Check sheet for the modelled part. Datum: model origin and axes. Units: mm. A direction names the side the tool comes from. Round coordinates to 2 decimals unless told otherwise and drop trailing zeros. Write each loop counter-clockwise with the first axis right and the second up, starting at its lowest first coordinate (ties: lowest second). Pieces come first, ordered by that corner, then holes.
Item 1: Depth check by flat-ended pin: pin 1 (12 mm diameter, centred on y = 15.5, z = 22.5, fed in from -X); pin 2 (8 mm diameter, centred on y = -33.5, z = 21, fed in from +X); pin 3 (3 mm diameter, centred on x = 19, y = 0.5, fed in from -Z). Enter the tip coordinate at first touch or a pass-through.
Item 2: Set-up check for faces 1 (the flat face through (-50, 35, 30)), 2 (the cylindrical face through (-27.5, 0.1, 4.9)), 3 (the cylindrical face through (-57.15, 36.99, 25.35)), 4 (the flat face through (-60, 0, 5)), 5 (the flat face through (-24, -1, 10)): record each of +Z, -Z, +X, -X, +Y, -Y from which the full face is reachable in a straight line by a thin tool's end or side.
Item 3: Section check A-A, the plane z = 35. State how many separate pieces and enclosed holes the cut face has, plus the area to 3 significant figures.
Item 4: Section check B-B, the plane x = -21.5. Record the cut outline in (y, z), plus the area to 3 significant figures.
Item 5: Section check C-C, the plane y = 0. Record the cut outline in (x, z).
Item 6: Release check for a two-part mould opening along Y. For faces 6 (the cylindrical face through (-57.15, -36.99, 25.35)), 7 (the flat face through (70, -1, 52)), 8 (the flat face through (-55, 30, 30)) record: pulls with the +Y half, pulls with the -Y half, needs draft (parallel to the pull), parting line crosses it, or undercut.
Item 7: Material ranges on line 1 along Z through (x, y) = (-19, -14); line 2 along Y through (x, z) = (-30, 8); line 3 along Z through (x, y) = (60.5, 37.5), recorded low to high.
Item 8: Section check D-D, the plane y = -36.5. Record the cut outline in (x, z).
from build123d import *

# Parameters (mm, degrees)
SALIENTE_EXTRUIR2_DEPTH = 50
CROQUIS4_W              = 140
CROQUIS4_H              = 100
SALIENTE_EXTRUIR3_DEPTH = 5
CROQUIS5_R              = 5
CORTAR_EXTRUIR1_DEPTH   = 5
CROQUIS6_W              = 50
CROQUIS6_H              = 40
CORTAR_EXTRUIR2_DEPTH   = 80
CROQUIS7_W              = 40
CROQUIS7_H              = 60
CORTAR_EXTRUIR3_DEPTH   = 50
CROQUIS8_R              = 2.5
CORTAR_EXTRUIR5_DEPTH   = 20
REDONDEO1_R             = 10
REDONDEO2_R             = 10
REDONDEO3_R             = 10
REDONDEO4_R             = 10


with BuildPart() as part:
    # Croquis1 → Saliente-Extruir2 (new body)
    with BuildSketch(Plane.XY):
        with BuildLine():
            Line((-60, 40), (-60, -40))
            Line((-60, -40), (20.000000086, -40))
            ThreePointArc((20.000000086, -40), (60, 8.6e-08), (19.999999914, 40))
            Line((19.999999914, 40), (-60, 40))
        make_face()
    extrude(amount=SALIENTE_EXTRUIR2_DEPTH)

    # Croquis4 → Saliente-Extruir3 (add)
    with BuildSketch(Plane.XY.offset(50)):
        Rectangle(CROQUIS4_W, CROQUIS4_H)
    extrude(amount=SALIENTE_EXTRUIR3_DEPTH)

    # Croquis5 → Cortar-Extruir1 (cut)
    with BuildSketch(Plane(origin=(0, 0, 0), x_dir=(-1, 0, 0), z_dir=(0, 0, -1))):
        with Locations((-20, 0)):
            Circle(CROQUIS5_R)
    extrude(amount=-CORTAR_EXTRUIR1_DEPTH, mode=Mode.SUBTRACT)

    # Croquis6 → Cortar-Extruir2 (cut)
    with BuildSketch(Plane(origin=(0, 40, 0), x_dir=(1, 0, 0), z_dir=(0, 1, 0))):
        with Locations((-25, -30)):
            Rectangle(CROQUIS6_W, CROQUIS6_H)
    extrude(amount=-CORTAR_EXTRUIR2_DEPTH, mode=Mode.SUBTRACT)

    # Croquis7 → Cortar-Extruir3 (cut)
    with BuildSketch(Plane.ZY.offset(60)):
        with Locations((30, 0)):
            Rectangle(CROQUIS7_W, CROQUIS7_H)
    extrude(amount=-CORTAR_EXTRUIR3_DEPTH, mode=Mode.SUBTRACT)

    # Croquis8 → Cortar-Extruir5 (cut)
    with BuildSketch(Plane(origin=(0, 0, 0), x_dir=(-1, 0, 0), z_dir=(0, 0, -1))):
        with Locations((30, 0)):
            Circle(CROQUIS8_R)
    extrude(amount=-CORTAR_EXTRUIR5_DEPTH, mode=Mode.SUBTRACT)

    # Redondeo1
    redondeo1_edges = [part.edges().sort_by_distance(p)[0] for p in [
        (70, -50, 52.5),
    ]]
    fillet(redondeo1_edges, radius=REDONDEO1_R)

    # Redondeo2
    redondeo2_edges = [part.edges().sort_by_distance(p)[0] for p in [
        (70, 50, 52.5),
    ]]
    fillet(redondeo2_edges, radius=REDONDEO2_R)

    # Redondeo3
    redondeo3_edges = [part.edges().sort_by_distance(p)[0] for p in [
        (-60, -40, 25),
    ]]
    fillet(redondeo3_edges, radius=REDONDEO3_R)

    # Redondeo4
    redondeo4_edges = [part.edges().sort_by_distance(p)[0] for p in [
        (-60, 40, 25),
    ]]
    fillet(redondeo4_edges, radius=REDONDEO4_R - 0.0001)  # a hair under: the kernel refuses the full size


solid = part.part
Values found:
1. pin 1: stops at x = 0
1. pin 2: stops at x = 47.01
1. pin 3: stops at z = 5
2. face 1: +Y, -Y
2. face 2: -Z
2. face 3: -Z, -X, +Y
2. face 4: -Z, -X, +Y, -Y
2. face 5: none
3. separate pieces: 3
3. enclosed holes: 0
3. area: 4,270 mm2
4. outline: (-50, 50) - (50, 50) - (50, 55) - (-50, 55) - close; (-40, 0) - (40, 0) - (40, 10) - (-40, 10) - close
4. area: 1,300 mm2
5. outline: (-70, 50) - (0, 50) - (0, 10) - (-27.5, 10) - (-27.5, 0) - (15, 0) - (15, 5) - (25, 5) - (25, 0) - (60, 0) - (60, 50) - (70, 50) - (70, 55) - (-70, 55) - close; (-60, 0) - (-32.5, 0) - (-32.5, 10) - (-60, 10) - close
6. face 6: pulls with the -Y half
6. face 7: needs draft
6. face 8: undercut
7. line 1: z = 0 to 10, 50 to 55
7. line 2: y = -40 to -2.5, 2.5 to 40
7. line 3: z = 50 to 55
8. outline: (-70, 50) - (-57.6, 50) - (-57.6, 0) - (36.36, 0) - (36.36, 50) - (70, 50) - (70, 55) - (-70, 55) - close; hole (-50, 10) - (0, 10) - (0, 50) - (-50, 50) - close
